Build history of the part. All positions in model axes, mm. Round coordinates to 2 decimals unless told otherwise and drop trailing zeros. Write each loop counter-clockwise with the first axis right and the second up, starting at its lowest first coordinate (ties: lowest second). Pieces come first, ordered by that corner, then holes.
Item 1: Band-saw the part on B-B, the plane x = 7.62. Write the cut outline in (y, z) (3 decimals), then the cut area to 3 significant figures.
Item 2: Band-saw the part on A-A, the plane z = -179.8. Write the cut outline in (x, y) (3 decimals).
Item 3: Band-saw the part on C-C, the plane z = -9.5. Write the cut outline in (x, y) (3 decimals).
Item 4: Wall check: probe 1 along X at (y, z) = (7, -350.1) (3 decimals); probe 2 along Z at (x, y) = (65.9, 3) (3 decimals); probe 3 along X at (y, z) = (3.5, -179.8) (3 decimals). Give the ranges that are in metal, low to high.
Item 5: Drop a flat-ended pin along its axis: pin 1 Ø5.5 at (x, z) = (7.62, -350.1) entering from -Y. Give the stop position or say it passes through.
Autodesk Inventor part; units mm, degrees
ref_plane "YZ Plane" through (0, 0, 0) normal (1, 0, 0) x (0, 1, 0)
ref_plane "XZ Plane" through (0, 0, 0) normal (0, 1, 0) x (-1, 0, 0)
ref_plane "XY Plane" through (0, 0, 0) normal (0, 0, 1) x (1, 0, 0)
sketch "Sketch1" plane through (0, 0, 0) normal (0, 1, 0) x (-1, 0, 0)
  line L0 (0, 0) -> (-78.2, 0)
  line L1 (-78.2, 0) -> (-78.2, -359.6)
  line L2 (-78.2, -359.6) -> (0, -359.6)
  line L3 (0, -359.6) -> (0, 0)
  dimension "d0" = 78.2
  dimension "d1" = 359.6
extrude "Extrusion1" add sketch "Sketch1" along normal blind 10
sketch "Sketch2" plane through (0, 0, 0) normal (0, -1, 0) x (1, 0, 0)
  circle A0 centre (7.62, -350.1) radius 3.175
  circle A1 centre (68.58, -350.1) radius 3.175
  circle A2 centre (7.62, -9.5) radius 3.175
  circle A3 centre (68.58, -9.5) radius 3.175
extrude "Extrusion2" cut sketch "Sketch2" against normal blind 25.4
sketch "Sketch3" plane through (0, 0, 0) normal (0, -1, 0) x (1, 0, 0)
  circle A0 centre (65.9, -179.8) radius 3.175
  dimension "d8" = 6.35
extrude "Extrusion3" cut sketch "Sketch3" against normal blind 25.4
properties part number "Top Plate" material "Aluminum 6061"
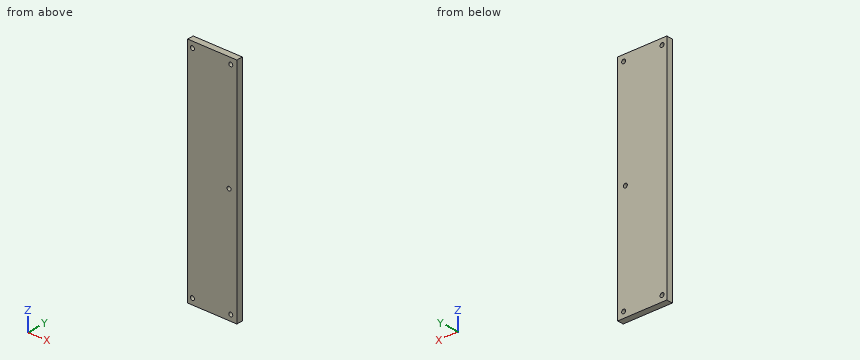
Results:
1. outline: (0, -359.6) - (10, -359.6) - (10, -353.275) - (0, -353.275) - close; (0, -346.925) - (10, -346.925) - (10, -12.675) - (0, -12.675) - close; (0, -6.325) - (10, -6.325) - (10, 0) - (0, 0) - close
1. area: 3,470 mm2
2. outline: (0, 0) - (62.725, 0) - (62.725, 10) - (0, 10) - close; (69.075, 0) - (78.2, 0) - (78.2, 10) - (69.075, 10) - close
3. outline: (0, 0) - (4.445, 0) - (4.445, 10) - (0, 10) - close; (10.795, 0) - (65.405, 0) - (65.405, 10) - (10.795, 10) - close; (71.755, 0) - (78.2, 0) - (78.2, 10) - (71.755, 10) - close
4. probe 1: x = 0 to 4.445, 10.795 to 65.405, 71.755 to 78.2
4. probe 2: z = -359.6 to -351.802, -348.398 to -182.975, -176.625 to -11.202, -7.798 to 0
4. probe 3: x = 0 to 62.725, 69.075 to 78.2
5. pin 1: passes through
